Verification items for the finished model (mm, model axes). Face numbers are marked on the shaded views. A direction names the side the tool comes from. Give positions to 0.01 mm unless a question says otherwise; leave off trailing zeros. Loops run counter-clockwise (first coordinate to the right, second up) from the corner with the lowest first, then second, coordinate; pieces in that order, holes last. Notation, with made-up numbers: (38, -27) - (83, -27) arc R28 cw to (83, -7) - close; hole circle Ø1 at (65, 62.5). An arc over 180 degrees is marked (long way). Use one line per item in the form item = value.
```python
from build123d import *

# Parameters (mm, degrees)
F0_R          = 20
F0_R_2        = 7.5
F1_DEPTH      = 30
F2_DEPTH      = 35
F2_DEPTH_BACK = 5
F4_R          = 7.5
F5_DEPTH      = 40.001
F6_R          = 1


with BuildPart() as f1:
    # F0 (on Front) → F1 (new body)
    with BuildSketch(Plane.XZ):
        Circle(F0_R)
        Circle(F0_R_2, mode=Mode.SUBTRACT)
    extrude(amount=F1_DEPTH)

    # F0 (on Front) → F2 (join, two sides)
    with BuildSketch(Plane.XZ) as f2_sk:
        Circle(F0_R_2)
    extrude(amount=F2_DEPTH)
    extrude(f2_sk.sketch, amount=-F2_DEPTH_BACK)

    # F4 (on offset) → F5 (cut, through all)
    with BuildSketch(Plane.YZ.offset(20)):
        with Locations((-15, 0)):
            Circle(F4_R)
    extrude(amount=-F5_DEPTH, mode=Mode.SUBTRACT)

    # F6
    f6_edges = [f1.edges().sort_by_distance(p)[0] for p in [
        (-20, -30, 0),
        (-20, 0, 0),
    ]]
    fillet(f6_edges, radius=F6_R)


solid = f1.part
```
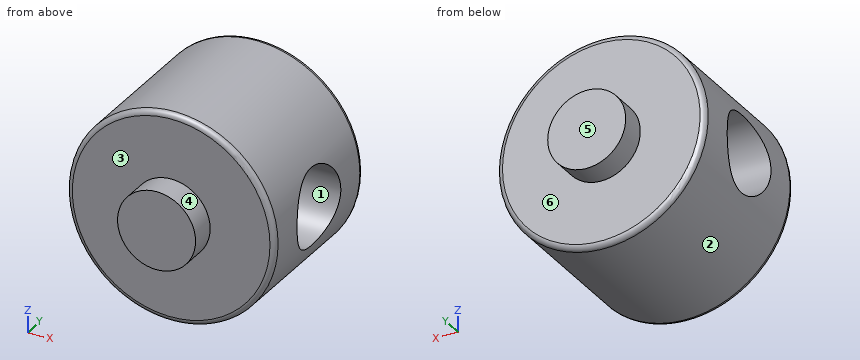
1. Tool access check on the marked faces 4, 5 and 6. Record the directions out of +Z, -Z, +X, -X, +Y, -Y that give a thin tool (end or side, any length) a straight path to the whole face; none if there is none.
Result set:
face_4 = -Y
face_5 = +Z, -Z, +X, -X, +Y
face_6 = +Y
2. Draft check along Z on the marked faces 1, 2 and 3. Enter one of: released by +Z, released by -Z, zero draft, split by the parting line, or undercut.
Result set:
face_1 = undercut
face_2 = split by the parting line
face_3 = zero draft
3. Scan lines: probe 1 along Y at (x, z) = (2, 0); probe 2 along Y at (x, z) = (14, -11.5); probe 3 along Z at (x, y) = (-5, -15). Record each from-to range of solid material in increasing order.
Result set:
probe_1 = -35 to -22.5, -7.5 to 5
probe_2 = -30 to 0
probe_3 = -19.36 to -7.5, 7.5 to 19.36
4. Depth check by flat-ended pin: pin 1 Ø3 at (x, y) = (2, -25.5) entering from -Z; pin 2 Ø3 at (x, y) = (4.5, -14.5) entering from -Z; pin 3 Ø1 at (y, z) = (-12.5, -12.5) entering from -X. Enter the tip coordinate at first touch or a pass-through.
Result set:
pin_1 = -19.99
pin_2 = -19.77
pin_3 = -16
5. Section check C-C, the plane y = -15. Record the cut outline in (x, z).
Result set:
outline = (-18.54, -7.5) arc R20 ccw to (18.54, -7.5) - close; (-18.54, 7.5) - (18.54, 7.5) arc R20 ccw to start
6. Section check A-A, the plane x = 0. Record the cut outline in (y, z), then the cut area to 3 significant figures.
Result set:
outline = (-35, -7.5) - (-30, -7.5) - (-30, -19) arc R1 ccw to (-29, -20) - (-1, -20) arc R1 ccw to (0, -19) - (0, -7.5) - (5, -7.5) - (5, 7.5) - (0, 7.5) - (0, 19) arc R1 ccw to (-1, 20) - (-29, 20) arc R1 ccw to (-30, 19) - (-30, 7.5) - (-35, 7.5) - close; hole circle Ø15 at (-15, 0)
area = 1,170 mm²
7. Section check D-D, the plane y = -25. Record the cut outline in (x, z).
Result set:
outline = circle Ø40 at (0, 0)
8. Section check B-B, the plane z = 0. Record the cut outline in (x, y), then the cut area to 3 significant figures.
Result set:
outline = (-20, -29) arc R1 ccw to (-19, -30) - (-7.5, -30) - (-7.5, -35) - (7.5, -35) - (7.5, -30) - (19, -30) arc R1 ccw to (20, -29) - (20, -22.5) - (-20, -22.5) - close; (-20, -7.5) - (20, -7.5) - (20, -1) arc R1 ccw to (19, 0) - (7.5, 0) - (7.5, 5) - (-7.5, 5) - (-7.5, 0) - (-19, 0) arc R1 ccw to (-20, -1) - close
area = 749 mm²
